```python
from build123d import *

# Parameters (mm, degrees)
SKETCH2_R           = 1.6
BOSS_EXTRUDE2_DEPTH = 7.5
SKETCH3_R           = 1.6
BOSS_EXTRUDE3_DEPTH = 7.5


with BuildPart() as part:
    # Sketch2 → Boss-Extrude2 (new body)
    with BuildSketch(Plane(origin=(0, 0, 0), x_dir=(1, 0, 0), z_dir=(0, 1, 0))):
        with BuildLine():
            Line((43.966606646, 5), (44.520107816, 5))
            ThreePointArc((44.520107816, 5), (44.8, 0), (44.520107816, -5))
            Line((44.520107816, -5), (43.966606646, -5))
            ThreePointArc((43.966606646, -5), (31.289475067, -31.289475068), (5, -43.966606646))
            Line((5, -43.966606646), (5, -44.520107816))
            ThreePointArc((5, -44.520107816), (0, -44.8), (-5, -44.520107816))
            Line((-5, -44.520107816), (-5, -43.966606646))
            ThreePointArc((-5, -43.966606646), (-31.289475068, -31.289475067), (-43.966606646, -5))
            Line((-43.966606646, -5), (-44.520107816, -5))
            ThreePointArc((-44.520107816, -5), (-44.8, 0), (-44.520107816, 5))
            Line((-44.520107816, 5), (-43.966606646, 5))
            ThreePointArc((-43.966606646, 5), (-31.289475067, 31.289475068), (-5, 43.966606646))
            Line((-5, 43.966606646), (-5, 44.520107816))
            ThreePointArc((-5, 44.520107816), (0, 44.8), (5, 44.520107816))
            Line((5, 44.520107816), (5, 43.966606646))
            ThreePointArc((5, 43.966606646), (31.289475068, 31.289475067), (43.966606646, 5))
        make_face()
        with Locations(Location((36.25, 0, 0), (0, 0, 270))):
            Circle(SKETCH2_R, mode=Mode.SUBTRACT)
        with Locations(Location((25.632620818, -25.632620818, 0), (0, 0, 270))):
            Circle(SKETCH2_R, mode=Mode.SUBTRACT)
        with Locations(Location((-36.25, 0, 0), (0, 0, 270))):
            Circle(SKETCH2_R, mode=Mode.SUBTRACT)
        with Locations(Location((-25.632620818, 25.632620818, 0), (0, 0, 270))):
            Circle(SKETCH2_R, mode=Mode.SUBTRACT)
        with Locations(Location((0, 36.25, 0), (0, 0, 270))):
            Circle(SKETCH2_R, mode=Mode.SUBTRACT)
        with Locations(Location((25.632620818, 25.632620818, 0), (0, 0, 270))):
            Circle(SKETCH2_R, mode=Mode.SUBTRACT)
        with BuildLine():
            Line((31.43, 3), (31.43, -3))
            ThreePointArc((31.43, -3), (32.015786437, -4.414213563), (33.43, -5))
            Line((33.43, -5), (36.58614437, -5))
            ThreePointArc((36.58614437, -5), (38.127674053, -5.725487102), (38.550739297, -7.375838913))
            ThreePointArc((38.550739297, -7.375838913), (36.262271651, -15.02032472), (32.474994889, -22.043983464))
            ThreePointArc((32.474994889, -22.043983464), (31.00886763, -22.911806118), (29.405844687, -22.334776876))
            Line((29.405844687, -22.334776876), (27.174113601, -20.103045789))
            ThreePointArc((27.174113601, -20.103045789), (25.759900039, -19.517259351), (24.345686476, -20.103045789))
            Line((24.345686476, -20.103045789), (20.103045789, -24.345686476))
            ThreePointArc((20.103045789, -24.345686476), (19.517259351, -25.759900039), (20.103045789, -27.174113601))
            Line((20.103045789, -27.174113601), (22.334776875, -29.405844688))
            ThreePointArc((22.334776875, -29.405844688), (22.911806119, -31.00886763), (22.043983464, -32.474994889))
            ThreePointArc((22.043983464, -32.474994889), (-15.02032472, -36.262271651), (-38.550739297, -7.375838914))
            ThreePointArc((-38.550739297, -7.375838914), (-38.127674054, -5.725487102), (-36.58614437, -5))
            Line((-36.58614437, -5), (-33.43, -5))
            ThreePointArc((-33.43, -5), (-32.015786438, -4.414213562), (-31.43, -3))
            Line((-31.43, -3), (-31.43, 3))
            ThreePointArc((-31.43, 3), (-32.015786437, 4.414213563), (-33.43, 5))
            Line((-33.43, 5), (-36.58614437, 5))
            ThreePointArc((-36.58614437, 5), (-38.127674053, 5.725487102), (-38.550739297, 7.375838913))
            ThreePointArc((-38.550739297, 7.375838913), (-36.262271651, 15.02032472), (-32.474994889, 22.043983464))
            ThreePointArc((-32.474994889, 22.043983464), (-31.00886763, 22.911806118), (-29.405844687, 22.334776876))
            Line((-29.405844687, 22.334776876), (-27.174113601, 20.103045789))
            ThreePointArc((-27.174113601, 20.103045789), (-25.759900039, 19.517259351), (-24.345686476, 20.103045789))
            Line((-24.345686476, 20.103045789), (-20.103045789, 24.345686476))
            ThreePointArc((-20.103045789, 24.345686476), (-19.517259351, 25.759900039), (-20.103045789, 27.174113601))
            Line((-20.103045789, 27.174113601), (-22.334776875, 29.405844688))
            ThreePointArc((-22.334776875, 29.405844688), (-22.911806119, 31.00886763), (-22.043983464, 32.474994889))
            ThreePointArc((-22.043983464, 32.474994889), (-15.020324721, 36.262271651), (-7.375838914, 38.550739297))
            ThreePointArc((-7.375838914, 38.550739297), (-5.725487102, 38.127674054), (-5, 36.58614437))
            Line((-5, 36.58614437), (-5, 33.43))
            ThreePointArc((-5, 33.43), (-4.414213562, 32.015786438), (-3, 31.43))
            Line((-3, 31.43), (3, 31.43))
            ThreePointArc((3, 31.43), (4.414213563, 32.015786437), (5, 33.43))
            Line((5, 33.43), (5, 36.58614437))
            ThreePointArc((5, 36.58614437), (5.725487102, 38.127674053), (7.375838913, 38.550739297))
            ThreePointArc((7.375838913, 38.550739297), (15.02032472, 36.262271651), (22.043983464, 32.474994889))
            ThreePointArc((22.043983464, 32.474994889), (22.911806118, 31.00886763), (22.334776876, 29.405844687))
            Line((22.334776876, 29.405844687), (20.103045789, 27.174113601))
            ThreePointArc((20.103045789, 27.174113601), (19.517259351, 25.759900039), (20.103045789, 24.345686476))
            Line((20.103045789, 24.345686476), (24.345686476, 20.103045789))
            ThreePointArc((24.345686476, 20.103045789), (25.759900039, 19.517259351), (27.174113601, 20.103045789))
            Line((27.174113601, 20.103045789), (29.405844688, 22.334776875))
            ThreePointArc((29.405844688, 22.334776875), (31.00886763, 22.911806119), (32.474994889, 22.043983464))
            ThreePointArc((32.474994889, 22.043983464), (36.262271651, 15.020324721), (38.550739297, 7.375838914))
            ThreePointArc((38.550739297, 7.375838914), (38.127674054, 5.725487102), (36.58614437, 5))
            Line((36.58614437, 5), (33.43, 5))
            ThreePointArc((33.43, 5), (32.015786438, 4.414213562), (31.43, 3))
        make_face(mode=Mode.SUBTRACT)
    extrude(amount=BOSS_EXTRUDE2_DEPTH)

    # Sketch3 → Boss-Extrude3 (add)
    with BuildSketch(Plane.XZ):
        with BuildLine():
            Line((22.440941356, -21.901962064), (-22.440941356, -21.901962064))
            Line((-22.440941356, -21.901962064), (-22.440941356, 6.65))
            Line((-22.440941356, 6.65), (-22.440941356, 11.341310409))
            ThreePointArc((-22.440941356, 11.341310409), (-23.026727793, 12.755523971), (-24.440941356, 13.341310409))
            Line((-24.440941356, 13.341310409), (-29.405844687, 13.341310409))
            Line((-29.405844687, 13.341310409), (-34.091425962, 13.341310409))
            ThreePointArc((-34.091425962, 13.341310409), (-35.536566009, 13.956827134), (-36.091425962, 15.426323995))
            Line((-36.091425962, 15.426323995), (-39.579540156, 15.426323995))
            Line((-39.579540156, 15.426323995), (-39.579540156, 13.341310409))
            Line((-39.579540156, 13.341310409), (-39.579540156, 3.405536176))
            Line((-39.579540156, 3.405536176), (-33.43, 3.405536176))
            Line((-33.43, 3.405536176), (-33.43, -5))
            Line((-33.43, -5), (-29.405844687, -5))
            Line((-29.405844687, -5), (-29.405844687, -22.334776876))
            Line((-29.405844687, -22.334776876), (-29.405844687, -29.405844688))
            Line((-29.405844687, -29.405844688), (-22.334776875, -29.405844688))
            Line((-22.334776875, -29.405844688), (22.334776876, -29.405844687))
            Line((22.334776876, -29.405844687), (29.405844688, -29.405844688))
            Line((29.405844688, -29.405844688), (29.405844688, -22.334776875))
            Line((29.405844688, -22.334776875), (29.405844687, 22.334776876))
            Line((29.405844687, 22.334776876), (29.405844688, 29.405844687))
            Line((29.405844688, 29.405844687), (23.434556913, 29.405844687))
            Line((23.434556913, 29.405844687), (23.434556913, 25.632620817))
            Line((23.434556913, 25.632620817), (22.440941356, 25.632620817))
            Line((22.440941356, 25.632620817), (22.440941356, 24.032620818))
            Line((22.440941356, 24.032620818), (22.440941356, -21.901962064))
        make_face()
        with Locations(Location((0, -26.847695671, 0), (0, 0, 270))):
            Circle(SKETCH3_R, mode=Mode.SUBTRACT)
        with Locations(Location((-25, 6.65, 0), (0, 0, 270))):
            Circle(SKETCH3_R, mode=Mode.SUBTRACT)
        with Locations(Location((25, 6.65, 0), (0, 0, 270))):
            Circle(SKETCH3_R, mode=Mode.SUBTRACT)
        with Locations(Location((25.632620818, 25.632620818, 0), (0, 0, 90))):
            Circle(SKETCH3_R, mode=Mode.SUBTRACT)
        with Locations(Location((-25.632620818, -25.632620818, 0), (0, 0, 90))):
            Circle(SKETCH3_R, mode=Mode.SUBTRACT)
        with Locations(Location((25.632620818, -25.632620818, 0), (0, 0, 90))):
            Circle(SKETCH3_R, mode=Mode.SUBTRACT)
    extrude(amount=-BOSS_EXTRUDE3_DEPTH)


solid = part.part
```
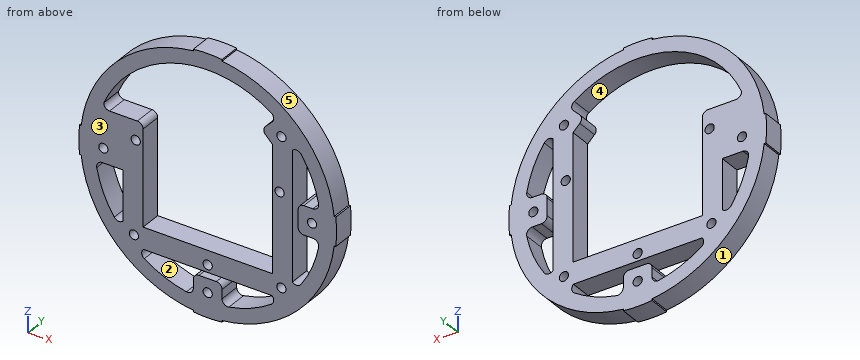
Verification items for the finished model (mm, model axes). Face numbers are marked on the shaded views. A direction names the side the tool comes from. Give positions to 0.01 mm unless a question says otherwise; leave off trailing zeros. Order: outer loops, then holes, each group sorted by start corner. A loop starts at its lowest first (then second) coordinate and runs counter-clockwise, first axis right, second up. Notation, with made-up numbers: M 76.5,50.5 L 83.5,50.5 A15 ccw 83.5,61.5 Z; hole C 45.5,29.25 d1. An arc over 180 degrees is marked long. Answer in a Markdown table with one row per item. Add a question column.
Item 1: Section check A-A, the plane z = 0. Enter the section's corners in (x, y), and give its area (3 significant figures).
Item 2: Section check B-B, the plane x = 0. Enter the section's corners in (y, z).
Item 3: Tool access check on the marked faces 1 and 2. Record the directions out of +Z, -Z, +X, -X, +Y, -Y that give a thin tool (end or side, any length) a straight path to the whole face; none if there is none.
Item 4: Scan lines: probe 1 along X at (y, z) = (2.75, 0); probe 2 along Z at (x, y) = (-7, 0.75); probe 3 along Z at (x, y) = (4.5, 5.75). Record each from-to range of solid material in increasing order. Write a range as from..to.
Item 5: Section check C-C, the plane y = 3.5. State how many separate pieces and enclosed holes the cut face has, and give its area (3 significant figures).
Item 6: Gauge pin test, flat ends, axial feed: pin 1 (1 mm diameter, centred on y = 3.5, z = 15, fed in from +X); pin 2 (3 mm diameter, centred on x = 28, y = 4, fed in from -Z); pin 3 (3.5 mm diameter, centred on x = 35, y = 4, fed in from -Z); pin 4 (6 mm diameter, centred on x = -32, z = -26.5, fed in from -Y). Record the tip position at first contact, or that the pin passes through.
Item 7: Mould release check, pull along X, two halves, no side actions. Record for the marked faces 3, 4 and 5: released by +X, released by -X, zero draft, split by the parting line, or undercut.
Filled sheet:
| question | item | result |
|---|---|---|
| 1 | outline | M -44.8,0 L -37.85,0 L -37.85,7.5 L -44.8,7.5 Z; M -34.65,0 L -22.44,0 L -22.44,7.5 L -34.65,7.5 Z; M 22.44,0 L 29.41,0 L 29.41,7.5 L 22.44,7.5 Z; M 31.43,0 L 34.65,0 L 34.65,7.5 L 31.43,7.5 Z; M 37.85,0 L 44.8,0 L 44.8,7.5 L 37.85,7.5 Z |
| 1 | area | 272 mm^2 |
| 2 | outline | M 0,-44.8 L 7.5,-44.8 L 7.5,-37.85 L 0,-37.85 Z; M 0,-34.65 L 7.5,-34.65 L 7.5,-31.43 L 0,-31.43 Z; M 0,-29.41 L 7.5,-29.41 L 7.5,-28.45 L 0,-28.45 Z; M 0,-25.25 L 7.5,-25.25 L 7.5,-21.9 L 0,-21.9 Z; M 0,39.25 L 7.5,39.25 L 7.5,44.8 L 0,44.8 Z |
| 3 | face 1 | -Z, -X, +Y, -Y |
| 3 | face 2 | +Y, -Y |
| 4 | probe 1 | x = -44.8..-37.85, -34.65..-22.44, 22.44..29.41, 31.43..34.65, 37.85..44.8 |
| 4 | probe 2 | z = -43.69..-38.59, -29.41..-21.9, 38.62..43.69 |
| 4 | probe 3 | z = -44.57..-32.11, -29.41..-21.9, 38.99..44.57 |
| 5 | separate pieces | 1 |
| 5 | enclosed holes | 13 |
| 5 | area | 2,660 mm^2 |
| 6 | pin 1 | stops at x = 41.81 |
| 6 | pin 2 | stops at z = -35.44 |
| 6 | pin 3 | stops at z = -29.2 |
| 6 | pin 4 | stops at y = 0 |
| 7 | face 3 | zero draft |
| 7 | face 4 | undercut |
| 7 | face 5 | released by +X |
